```python
from build123d import *

# Parameters (mm, degrees)
SKETCH1_W           = 123.825
SKETCH1_H           = 200.025
BOSS_EXTRUDE1_DEPTH = 6.35
CUT_EXTRUDE1_DEPTH  = 1
SKETCH3_R           = 3.175
CUT_EXTRUDE5_DEPTH  = 6.35


with BuildPart() as part:
    # Sketch1 → Boss-Extrude1 (new body)
    with BuildSketch(Plane.XY):
        with Locations((0, 100.0125)):
            Rectangle(SKETCH1_W, SKETCH1_H)
    extrude(amount=BOSS_EXTRUDE1_DEPTH)

    # Sketch2 → Cut-Extrude1 (cut)
    with BuildSketch(Plane.XY.offset(6.35)):
        with BuildLine():
            add(Edge.make_bspline(
                [(-9.3315137, 169.569243245), (-11.197682458, 168.0976913), (-14.473708818, 165.721233019), (-17.3515287, 161.55448265), (-18.744772102, 157.97825035), (-19.57008031, 154.001795446), (-19.358235831, 149.934925708), (-18.469822241, 146.12187465), (-17.124182712, 143.444668775), (-15.644034584, 140.599586864), (-13.588642306, 138.679050764), (-11.836257338, 136.982177805), (-10.077256706, 135.678856281), (-7.853613512, 134.599615465), (-5.185304822, 133.61558172), (-2.047786445, 132.897639564), (1.519421734, 132.841261276), (5.39237554, 133.515486042), (8.762284385, 135.063456784), (13.159045788, 137.534995882), (15.41933096, 140.673664776), (17.148115982, 142.599332984)],
                knots=[0, 0, 0, 0, 0.099961909, 0.167105029, 0.208449478, 0.26000516, 0.335840189, 0.376754282, 0.422870274, 0.460837159, 0.509980806, 0.539098001, 0.563057055, 0.601178667, 0.642018306, 0.681938728, 0.735202325, 0.790245849, 0.844804461, 0.889640513, 1, 1, 1, 1], degree=3))
            add(Edge.make_bspline(
                [(17.148115982, 142.599332984), (17.367564898, 144.13870869), (16.733511702, 146.581109303), (16.27851799, 149.765590012), (15.257046991, 151.728449354), (14.513019179, 153.196973861), (13.240823028, 154.375565069), (11.745568369, 155.781281157), (9.683821258, 156.19357481), (7.817396792, 156.396871018), (6.203806641, 155.97816213), (4.652965895, 155.265249531), (3.330558451, 154.147368605), (2.264943334, 152.806256443), (1.516548282, 151.083064738), (1.371346174, 147.894578102), (1.84694368, 145.341424214), (2.595738039, 143.569491513)],
                knots=[0, 0, 0, 0, 0.129227486, 0.217526215, 0.272879708, 0.318699717, 0.357375737, 0.421225341, 0.491051763, 0.532380112, 0.58197413, 0.631697637, 0.678188113, 0.729298629, 0.777918757, 0.836782647, 1, 1, 1, 1], degree=3))
            add(Edge.make_bspline(
                [(2.595738039, 143.569491513), (1.091260425, 144.310158379), (-0.219261636, 146.215388888), (-1.583212927, 149.064413701), (-2.047008332, 151.87724563), (-1.347571294, 155.191523623), (0.573453598, 158.349369243), (2.984260186, 160.391278639), (6.053225923, 162.32432944), (9.778943871, 162.556297831), (14.026176553, 162.441587138), (17.093369221, 160.81063786), (19.954602244, 158.976975505), (21.782777067, 156.302763768), (23.650890625, 153.012737551), (25.241855425, 147.240745591), (25.735418593, 140.388419647), (24.627732078, 133.63565983), (23.078571098, 129.062371922), (21.165081325, 125.256739903), (18.863141262, 122.066101255), (16.769401407, 119.576261489), (14.765247422, 117.697271946), (12.495470846, 115.768794509), (9.628425201, 114.075558071), (6.510664621, 112.417594108), (3.292717559, 111.195822905), (-0.597926715, 110.157178984), (-5.997823526, 109.821254189), (-10.108137267, 110.358818405), (-12.480099704, 111.116416453)],
                knots=[0, 0, 0, 0, 0.042580268, 0.060224686, 0.08386458, 0.116965183, 0.148096973, 0.180452989, 0.200374999, 0.24344269, 0.276533285, 0.312238472, 0.333844074, 0.366401949, 0.396661336, 0.434486559, 0.524427596, 0.57712071, 0.615572447, 0.652537223, 0.689999449, 0.720028669, 0.738935019, 0.763057377, 0.799114426, 0.827221945, 0.85696418, 0.890507339, 0.9340038, 1, 1, 1, 1], degree=3))
            add(Edge.make_bspline(
                [(-12.480099704, 111.116416453), (-10.129509341, 110.851795977), (-6.766504791, 111.676958112), (-1.98778411, 112.975517751), (2.16491123, 115.032216309), (6.576646899, 117.974608303), (9.964617235, 122.001460334), (13.774755311, 126.773576412), (15.547642905, 130.861311443), (16.02148027, 133.6801336)],
                knots=[0, 0, 0, 0, 0.176744277, 0.265013981, 0.379273682, 0.53095193, 0.667955404, 0.780622384, 1, 1, 1, 1], degree=3))
            add(Edge.make_bspline(
                [(16.02148027, 133.6801336), (15.284751167, 132.546381486), (13.729522727, 131.07018515), (11.664732098, 129.010614657), (9.597669158, 127.664469948), (7.112988668, 126.179760231), (3.800643978, 124.813352957), (0.241003836, 124.010205105), (-4.0915461, 123.798546407), (-9.411378564, 124.519214898), (-14.89887892, 127.064106493), (-19.214250688, 130.610000296), (-21.908165408, 134.091041706), (-25.432890172, 140.742158426), (-25.903440928, 149.142146476), (-23.050507432, 157.045363775), (-19.622590138, 162.033808821), (-15.135925354, 166.48695288), (-11.34416307, 168.928938218), (-9.3315137, 169.569243245)],
                knots=[0, 0, 0, 0, 0.046226378, 0.074002645, 0.100379959, 0.131070976, 0.173920494, 0.22349156, 0.256215817, 0.323367781, 0.406730252, 0.461306621, 0.514924876, 0.557488619, 0.720548112, 0.782951714, 0.845978771, 0.927692708, 1, 1, 1, 1], degree=3))
        make_face()
    extrude(amount=-CUT_EXTRUDE1_DEPTH, mode=Mode.SUBTRACT)

    # Sketch3 → Cut-Extrude5 (cut)
    with BuildSketch(Plane.XY):
        with Locations((49.2125, 88.9)):
            Circle(SKETCH3_R)
    extrude(amount=CUT_EXTRUDE5_DEPTH, mode=Mode.SUBTRACT)


solid = part.part
```
Source: CAD feature listing. Evaluate the final solid. Frame: model axes, mm. A direction names the side the tool comes from. Coordinates: 2 decimals unless noted, no trailing zeros. Loops run counter-clockwise (first coordinate to the right, second up) from the corner with the lowest first, then second, coordinate; pieces in that order, holes last. Notation, with made-up numbers: (-16.75, -7) - (-1.75, -7) arc R13 cw to (-1.75, 1) - close; hole circle Ø7 at (21.25, -28). An arc over 180 degrees is marked (long way). Answer as CSV lines item,"result".
1. Mould query, pull axis X, two halves, no side actions, for faces 3 (the flat face through (61.912, 99, 3)), 4 (the flat face through (-1, 0, 3)), 5 (the cylindrical face through (48.52, 85.8, 3.13)). Classes: released by +X, released by -X, zero draft, split by the parting line, or undercut.
Established:
face 3,"released by +X"
face 4,"zero draft"
face 5,"undercut"
2. Section A-A (y = 88.9). Return loops of the section in (x, z).
Established:
outline,"(-61.91, 0) - (46.04, 0) - (46.04, 6.35) - (-61.91, 6.35) - close; (52.39, 0) - (61.91, 0) - (61.91, 6.35) - (52.39, 6.35) - close"
3. Reachability of faces 1 (the flat face through (6, 133, 5.35)), 2 (the flat face through (-1, 200.025, 3)) from +Z, -Z, +X, -X, +Y, -Y: full face, straight path, thin tool, end or side. Return the list, or none.
Established:
face 1,"+Z"
face 2,"+Z, -Z, +X, -X, +Y"
4. Ray query, line 1 (Y direction, x = 47.5, z = 4.75) (3 decimals); line 2 (X direction, y = 129, z = 6); line 3 (X direction, y = 90, z = 2). Return the intervals inside material, ascending.
Established:
line 1,"y = 0 to 86.226, 91.574 to 200.025"
line 2,"x = -61.91 to -17.19, 11.52 to 14.58, 22.95 to 61.91"
line 3,"x = -61.91 to 46.23, 52.19 to 61.91"
